```python
from build123d import *

# Parameters (mm, degrees)
F0_R     = 16.5
F0_R_2   = 14.5
F1_DEPTH = 120
F2_R     = 14.5
F3_DEPTH = 5
F5_R     = 5
F6_R     = 1
F4_R     = 3.175
F7_DEPTH = 25


with BuildPart() as f1:
    # F0 (on Top) → F1 (new body)
    with BuildSketch(Plane.XY):
        Circle(F0_R)
        Circle(F0_R_2, mode=Mode.SUBTRACT)
    extrude(amount=F1_DEPTH)

    # F2 (on face) → F3 (join)
    with BuildSketch(Plane.XY.offset(120)):
        Circle(F2_R)
    extrude(amount=-F3_DEPTH)

    # F5
    f5_edges = [f1.edges().sort_by_distance(p)[0] for p in [
        (-16.5, 0, 120),
    ]]
    fillet(f5_edges, radius=F5_R)

    # F6
    f6_edges = [f1.edges().sort_by_distance(p)[0] for p in [
        (-16.5, 0, 0),
    ]]
    fillet(f6_edges, radius=F6_R)

    # F4 (on face) → F7 (cut)
    with BuildSketch(Plane.XY.offset(120)):
        Circle(F4_R)
    extrude(amount=-F7_DEPTH, mode=Mode.SUBTRACT)


solid = f1.part
```
Here's how the part is built. I have some questions about the finished solid (model axes, mm). A direction names the side the tool comes from. Coordinates: 2 decimals unless noted, no trailing zeros. Order: outer loops, then holes, each group sorted by start corner. A loop starts at its lowest first (then second) coordinate and runs counter-clockwise, first axis right, second up.
Item 1: If we section it at C-C, the plane z = 88: List the corners of the cut face in (x, y) for me.
Response values:
outline: circle Ø33 at (0, 0); hole circle Ø29 at (0, 0)
Item 2: I need wall thicknesses on probe 1 along Y at (x, z) = (0, 89); probe 2 along Z at (x, y) = (11, -4); probe 3 along X at (y, z) = (-11, 64.5). Which ranges of each line are inside material? Lowest first, please.
Response values:
probe 1: y = -16.5 to -14.5, 14.5 to 16.5
probe 2: z = 115 to 120
probe 3: x = -12.3 to -9.45, 9.45 to 12.3
Item 3: Thinking about a two-plate mould opening in X: for faces 3 (the face through (6, -14, 0)), 4 (the face through (15.24, -6.32, 57.2)), 5 (the face through (-0.69, -3.1, 117.54)), which applies, pulls with the +X half, pulls with the -X half, needs draft (parallel to the pull), parting line crosses it, or undercut?
Response values:
face 3: needs draft
face 4: parting line crosses it
face 5: undercut
Item 4: If we section it at A-A, the plane x = 0: List the corners of the cut face in (y, z) for me (3 decimals), then the cut area to 3 significant figures.
Response values:
outline: (-16.5, 1) arc R1 ccw to (-15.5, 0) - (-14.5, 0) - (-14.5, 115) - (-3.175, 115) - (-3.175, 120) - (-11.5, 120) arc R5 ccw to (-16.5, 115) - close; (3.175, 115) - (14.5, 115) - (14.5, 0) - (15.5, 0) arc R1 ccw to (16.5, 1) - (16.5, 115) arc R5 ccw to (11.5, 120) - (3.175, 120) - close
area: 582 mm2
Item 5: Which directions (+Z, -Z, +X, -X, +Y, -Y) give clear straight access to the entire face, cutting with the end or side of a thin tool? Please do faces 1 (the face through (6.691, -12.864, 56.695)), 2 (the face through (2.4, -2.4, 120)).
Response values:
face 1: -Z
face 2: +Z, +X, -X, +Y, -Y
Item 6: I'm going to push flat-ended pins straight in: pin 1 Ø2 at (x, z) = (-7.5, 38.5) entering from -Y; pin 2 Ø1 at (x, z) = (-9, 25.5) entering from -Y; pin 3 Ø5 at (x, y) = (0, 0) entering from +Z; pin 4 Ø1.5 at (x, z) = (-10.5, 13.5) entering from -Y. Where does each tip first touch, or does it pass through?
Response values:
pin 1: stops at y = -15.17
pin 2: stops at y = -14.14
pin 3: passes through
pin 4: stops at y = -13.31
